The listing builds one solid part. Answer for the finished solid, in the listing's coordinates (mm). Coordinates: 2 decimals unless noted, no trailing zeros. Loops run counter-clockwise (first coordinate to the right, second up) from the corner with the lowest first, then second, coordinate; pieces in that order, holes last. Notation, with made-up numbers: (75, 84.25) -> (103, 84.25) arc R29 ccw to (103, 108.25) -> close; hole circle Ø9 at (-24.75, 17). An arc over 180 degrees is marked (long way). Answer in a Markdown table with one row per item.
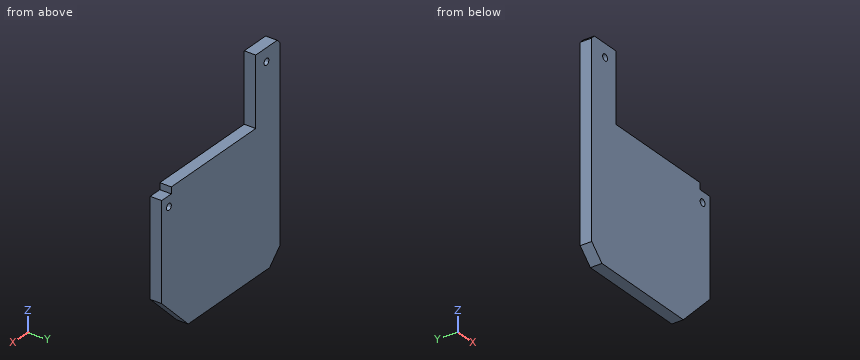
```python
from build123d import *

# Parameters (mm, degrees)
SKETCH1_W                = 42.3
SKETCH1_H                = 42.3
BOSS_EXTRUDE1_DEPTH      = 3.5
CUT_EXTRUDE1_DEPTH       = 3.5
CIRPATTERN1_COUNT        = 4
SKETCH5_W                = 42.3
SKETCH5_H                = 3.5
BOSS_EXTRUDE3_DEPTH      = 6.79
BOSS_EXTRUDE3_DEPTH_BACK = 6.79
CUT_EXTRUDE2_REACH       = 5.5
SKETCH6_W                = 4
SKETCH6_H                = 2
BOSS_EXTRUDE4_DEPTH      = 3.5
CHAMFER1_SIZE            = 1.1
SKETCH8_R                = 1
CUT_EXTRUDE3_DEPTH       = 3.5
CHAMFER2_SIZE            = 11
SKETCH10_R               = 1
CUT_EXTRUDE4_DEPTH       = 3.5


with BuildPart() as part:
    # Sketch1 → Boss-Extrude1 (new body)
    with BuildSketch(Plane(origin=(0, 0, 0), x_dir=(1, 0, 0), z_dir=(0, 1, 0))):
        Rectangle(SKETCH1_W, SKETCH1_H)
    extrude(amount=BOSS_EXTRUDE1_DEPTH)

    # Sketch2 → Cut-Extrude1 (cut)
    with BuildSketch(Plane(origin=(0, 3.5, 0), x_dir=(1, 0, 0), z_dir=(0, 1, 0))):
        Polygon((-21.15, 16.907359313), (-16.907359313, 21.15), (-21.15, 21.15), align=None)
    cut_extrude1 = extrude(amount=-CUT_EXTRUDE1_DEPTH, mode=Mode.SUBTRACT)

    # CirPattern1: Cut-Extrude1 ×4 about axis
    cirpattern1_axis = Axis((0, 0, 0), (0, 1, 0))
    for i in range(1, CIRPATTERN1_COUNT):
        add(cut_extrude1.rotate(cirpattern1_axis, i * 360 / CIRPATTERN1_COUNT), mode=Mode.SUBTRACT)

    # Sketch5 → Boss-Extrude3 (add, two sides)
    with BuildSketch(Plane(origin=(21.15, 0, 0), x_dir=(0, 0, -1), z_dir=(1, 0, 0))) as boss_extrude3_sk:
        with Locations((0, 1.75)):
            Rectangle(SKETCH5_W, SKETCH5_H)
    extrude(amount=BOSS_EXTRUDE3_DEPTH)
    extrude(boss_extrude3_sk.sketch, amount=-BOSS_EXTRUDE3_DEPTH_BACK)

    # Sketch6 → Cut-Extrude2 (cut, up to next)
    with BuildSketch(Plane(origin=(0, 3.5, 0), x_dir=(1, 0, 0), z_dir=(0, 1, 0)), mode=Mode.PRIVATE) as cut_extrude2_sk1:
        with Locations((25.94, -20.15)):
            Rectangle(SKETCH6_W, SKETCH6_H)
    cut_extrude2_tool1 = extrude(cut_extrude2_sk1.sketch, amount=-CUT_EXTRUDE2_REACH, mode=Mode.PRIVATE) & part.part
    add(cut_extrude2_tool1.solids().sort_by_distance((25.94, 3.5, 20.15))[0], mode=Mode.SUBTRACT)

    # Sketch7 → Boss-Extrude4 (add)
    with BuildSketch(Plane(origin=(0, 3.5, 0), x_dir=(1, 0, 0), z_dir=(0, 1, 0))):
        Polygon((-21.15, -16.907359313), (-21.15, -42.036504825), (-11.15, -42.036504825), (-11.15, -21.15), (-16.907359313, -21.15), align=None)
    extrude(amount=-BOSS_EXTRUDE4_DEPTH)

    # Chamfer1
    chamfer1_edges = [part.edges().sort_by_distance(p)[0] for p in [
        (-21.15, 1.75, 42.036504825),
    ]]
    chamfer(chamfer1_edges, length=CHAMFER1_SIZE)

    # Sketch8 → Cut-Extrude3 (cut)
    with BuildSketch(Plane.XZ):
        with Locations((-15.6, 38.036504825)):
            Circle(SKETCH8_R)
    extrude(amount=-CUT_EXTRUDE3_DEPTH, mode=Mode.SUBTRACT)

    # Chamfer2
    chamfer2_edges = [part.edges().sort_by_distance(p)[0] for p in [
        (27.94, 1.75, -21.15),
    ]]
    chamfer(chamfer2_edges, length=CHAMFER2_SIZE)

    # Sketch10 → Cut-Extrude4 (cut)
    with BuildSketch(Plane.XZ):
        with Locations((24.94, 15.956504825)):
            Circle(SKETCH10_R)
    extrude(amount=-CUT_EXTRUDE4_DEPTH, mode=Mode.SUBTRACT)


solid = part.part
```
Item 1: Flat-ended cylindrical pins translate along their axes: pin 1 Ø1.8 at (y, z) = (1, 35) entering from +X; pin 2 Ø1.2 at (x, z) = (24.94, 15.96) entering from +Y. Find the tip coordinate at first contact, or state that the pin passes through.
Findings below:
| item | result |
|---|---|
| pin 1 | stops at x = -11.15 |
| pin 2 | passes through |
Item 2: A cutting plane is placed at D-D, the plane z = 32. Determine the outline of the cut face in (x, y), plus the area to 3 significant figures.
Findings below:
| item | result |
|---|---|
| outline | (-21.15, 0) -> (-11.15, 0) -> (-11.15, 3.5) -> (-21.15, 3.5) -> close |
| area | 35.0 mm2 |
Item 3: A cutting plane is placed at A-A, the plane x = -15.6. Determine the outline of the cut face in (y, z), plus the area to 3 significant figures.
Findings below:
| item | result |
|---|---|
| outline | (0, -21.15) -> (3.5, -21.15) -> (3.5, 37.04) -> (0, 37.04) -> close; (0, 39.04) -> (3.5, 39.04) -> (3.5, 42.04) -> (0, 42.04) -> close |
| area | 214 mm2 |
Item 4: A cutting plane is placed at C-C, the plane x = 24.94. Determine the outline of the cut face in (y, z).
Findings below:
| item | result |
|---|---|
| outline | (0, -13.15) -> (3.5, -13.15) -> (3.5, 14.96) -> (0, 14.96) -> close; (0, 16.96) -> (3.5, 16.96) -> (3.5, 19.15) -> (0, 19.15) -> close |
Item 5: A cutting plane is placed at B-B, the plane y = 2. Determine the outline of the cut face in (x, z), plus the area to 3 significant figures.
Findings below:
| item | result |
|---|---|
| outline | (-21.15, -16.91) -> (-16.91, -21.15) -> (16.94, -21.15) -> (27.94, -10.15) -> (27.94, 19.15) -> (23.94, 19.15) -> (23.94, 21.15) -> (-11.15, 21.15) -> (-11.15, 42.04) -> (-20.05, 42.04) -> (-21.15, 40.94) -> close; hole circle Ø2 at (-15.6, 38.04); hole circle Ø2 at (24.94, 15.96) |
| area | 2,200 mm2 |
Item 6: Find the intervals of material crossed by probe 1 along Z at (x, y) = (-15.6, 2); probe 2 along X at (y, z) = (2.3, 31); probe 3 along Z at (x, y) = (13, 1.9), in increasing order.
Findings below:
| item | result |
|---|---|
| probe 1 | z = -21.15 to 37.04, 39.04 to 42.04 |
| probe 2 | x = -21.15 to -11.15 |
| probe 3 | z = -21.15 to 21.15 |
